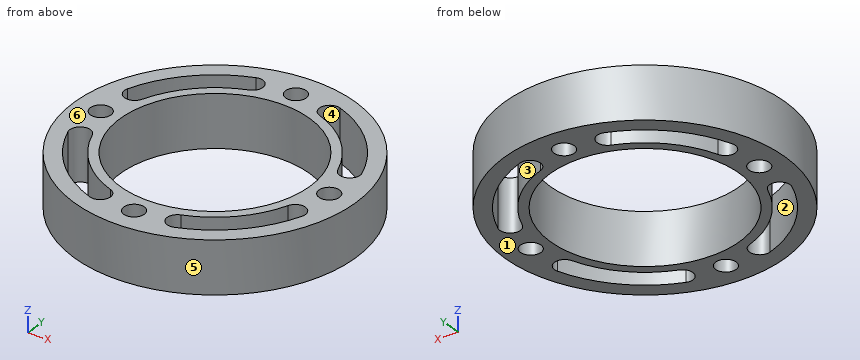
from build123d import *

# Parameters (mm, degrees)
SKETCH_1_R      = 21.5
SKETCH_1_R_2    = 14.5
SKETCH_1_R_3    = 1.575
EXTRUDE_1_DEPTH = 8


with BuildPart() as part:
    # 草图1 → 凸台-拉伸1 (new body)
    with BuildSketch(Plane.XY):
        Circle(SKETCH_1_R)
        Circle(SKETCH_1_R_2, mode=Mode.SUBTRACT)
        with Locations((0, 17.5)):
            Circle(SKETCH_1_R_3, mode=Mode.SUBTRACT)
        with Locations((17.5, 0)):
            Circle(SKETCH_1_R_3, mode=Mode.SUBTRACT)
        with Locations((0, -17.5)):
            Circle(SKETCH_1_R_3, mode=Mode.SUBTRACT)
        with Locations((-17.5, 0)):
            Circle(SKETCH_1_R_3, mode=Mode.SUBTRACT)
        with BuildLine():
            ThreePointArc((-5.379173171, 14.989), (-4.428750737, 17.003434709), (-6.443185446, 17.953857143))
            ThreePointArc((-6.443185446, 17.953857143), (-13.488061851, 13.488061851), (-17.953857143, 6.443185446))
            ThreePointArc((-17.953857143, 6.443185446), (-17.003434709, 4.428750737), (-14.989, 5.379173171))
            ThreePointArc((-14.989, 5.379173171), (-11.26067549, 11.26067549), (-5.379173171, 14.989))
        make_face(mode=Mode.SUBTRACT)
        with BuildLine():
            ThreePointArc((5.379173171, 14.989), (11.26067549, 11.26067549), (14.989, 5.379173171))
            ThreePointArc((14.989, 5.379173171), (17.003434709, 4.428750737), (17.953857143, 6.443185446))
            ThreePointArc((17.953857143, 6.443185446), (13.488061851, 13.488061851), (6.443185446, 17.953857143))
            ThreePointArc((6.443185446, 17.953857143), (4.428750737, 17.003434709), (5.379173171, 14.989))
        make_face(mode=Mode.SUBTRACT)
        with BuildLine():
            ThreePointArc((5.379173171, -14.989), (4.428750737, -17.003434709), (6.443185446, -17.953857143))
            ThreePointArc((6.443185446, -17.953857143), (13.488061851, -13.488061851), (17.953857143, -6.443185446))
            ThreePointArc((17.953857143, -6.443185446), (17.003434709, -4.428750737), (14.989, -5.379173171))
            ThreePointArc((14.989, -5.379173171), (11.26067549, -11.26067549), (5.379173171, -14.989))
        make_face(mode=Mode.SUBTRACT)
        with BuildLine():
            ThreePointArc((-5.379173171, -14.989), (-11.26067549, -11.26067549), (-14.989, -5.379173171))
            ThreePointArc((-14.989, -5.379173171), (-17.003434709, -4.428750737), (-17.953857143, -6.443185446))
            ThreePointArc((-17.953857143, -6.443185446), (-13.488061851, -13.488061851), (-6.443185446, -17.953857143))
            ThreePointArc((-6.443185446, -17.953857143), (-4.428750737, -17.003434709), (-5.379173171, -14.989))
        make_face(mode=Mode.SUBTRACT)
    extrude(amount=EXTRUDE_1_DEPTH)


solid = part.part
Could you check a few things on this model? Use its own coordinates, in mm. Face numbers are marked on the shaded views. A direction names the side the tool comes from. Give positions to 0.01 mm unless a question says otherwise; leave off trailing zeros. Order: outer loops, then holes, each group sorted by start corner. A loop starts at its lowest first (then second) coordinate and runs counter-clockwise, first axis right, second up. Notation, with made-up numbers: (21, 29.5) - (33, 29.5) arc R11 cw to (33, 42.5) - close; hole circle Ø3 at (-7, 47). An arc over 180 degrees is marked (long way). Return JSON: item names as keys, results as strings. Group by question number.
Q1. Thinking about a two-plate mould opening in Y: for the marked faces 3, 4, 5 and 6, which applies, pulls with the +Y half, pulls with the -Y half, needs draft (parallel to the pull), parting line crosses it, or undercut?
Q2. Please list where these lines run through material, in increasing order: line 1 along Y through (x, z) = (0, 3) (3 decimals); line 2 along X through (y, z) = (-10.5, 1.75) (3 decimals); line 3 along Y through (x, z) = (17.5, 6) (3 decimals). Write a range as [from, to].
Q3. Which directions (+Z, -Z, +X, -X, +Y, -Y) give clear straight access to the entire face, cutting with the end or side of a thin tool? Please do the marked faces 1 and 2.
Q4. Suppose I cut it at C-C, the plane z = 2. State how many separate pieces and enclosed holes the cut face has, and give its area (3 significant figures).
Q5. Suppose I cut it at A-A, the plane x = 0. Please give me the cut outline in (y, z) (3 decimals), and give its area (3 significant figures).
Q6. Will these pins go through, and if not, where does the flat tip stop? pin 1 Ø1 at (x, y) = (-6, -15.5) entering from +Z; pin 2 Ø4 at (x, z) = (10.5, 3.5) entering from +Y; pin 3 Ø1.5 at (x, z) = (-16, 5) entering from +Y.
Resolved:
{
 "1": {"face 3": "undercut", "face 4": "undercut", "face 5": "parting line crosses it", "face 6": "needs draft"},
 "2": {"line 1": "y = [-21.5, -19.075], [-15.925, -14.5], [14.5, 15.925], [19.075, 21.5]", "line 2": "x = [-18.762, -15.925], [-11.973, -10], [10, 11.973], [15.925, 18.762]", "line 3": "y = [-12.49, -7.59], [-4.718, -1.575], [1.575, 4.718], [7.59, 12.49]"},
 "3": {"face 1": "-Z, +X, -X, +Y, -Y", "face 2": "+Z, -Z"},
 "4": {"separate pieces": "1", "enclosed holes": "9", "area": "535 mm2"},
 "5": {"outline": "(-21.5, 0) - (-19.075, 0) - (-19.075, 8) - (-21.5, 8) - close; (-15.925, 0) - (-14.5, 0) - (-14.5, 8) - (-15.925, 8) - close; (14.5, 0) - (15.925, 0) - (15.925, 8) - (14.5, 8) - close; (19.075, 0) - (21.5, 0) - (21.5, 8) - (19.075, 8) - close", "area": "61.6 mm2"},
 "6": {"pin 1": "passes through", "pin 2": "stops at y = 19.75", "pin 3": "stops at y = 15.16"}
}
